from build123d import *

# Parameters (mm, degrees)
F2_DEPTH       = 20
F4_D           = 4
F4_CSINK_D     = 8
F4_CSINK_ANGLE = 90
F6_W           = 8
F6_H           = 2
F7_DEPTH       = 16.001


with BuildPart() as f2:
    # F1 (on Right) → F2 (new body, symmetric)
    with BuildSketch(Plane.YZ):
        Polygon((-16, 0), (0, 0), (0, 16), align=None)
    extrude(amount=F2_DEPTH, both=True)

    # F4 (through all)
    with Locations(Plane(origin=(0, -8, 8), x_dir=(1, 0, 0), z_dir=(0, -0.7071067812, 0.7071067812))):
        with Locations((-12, 0)):
            CounterSinkHole(F4_D / 2, F4_CSINK_D / 2, counter_sink_angle=F4_CSINK_ANGLE)

    # F5: F2 across plane


with BuildPart() as f2_1:
    add(f2.part)
    add(f2.part.mirror(Plane.YZ), mode=Mode.INTERSECT)

    # F6 (on face) → F7 (cut, through all)
    with BuildSketch(Plane(origin=(0, 0, 0), x_dir=(1, 0, 0), z_dir=(0, 0, -1))):
        with Locations((0, 1)):
            Rectangle(F6_W, F6_H)
    extrude(amount=-F7_DEPTH, mode=Mode.SUBTRACT)


solid = f2_1.part
Verification items for the finished model (mm, model axes). A direction names the side the tool comes from. Coordinates: 2 decimals unless noted, no trailing zeros. Order: outer loops, then holes, each group sorted by start corner. A loop starts at its lowest first (then second) coordinate and runs counter-clockwise, first axis right, second up. Notation, with made-up numbers: M 85.25,-25.5 L 128.25,-25.5 A25 cw 128.25,7.5 Z; hole C 42.25,64.25 d9. An arc over 180 degrees is marked long. One line per item, written item: value. Start each with the question number.
Item 1: Sectioned sample at A-A (z = 15). Enter the section's corners in (x, y), then the cut area to 3 significant figures.
Item 2: Access from +Z, -Z, +X, -X, +Y, -Y to the whole of each face (thin tool, end or side, straight path). Record for faces 1 (the flat face through (20, -5, 5)), 2 (the flat face through (4, -1, 8)).
Item 3: Sectioned sample at C-C (x = -12). Enter the section's corners in (y, z).
Item 4: Sectioned sample at B-B (z = 13.25). Enter the section's corners in (x, y).
Item 5: Mould release check, pull along X, two halves, no side actions. Record for faces 3 (the flat face through (12, 0, 8)), 4 (the cylindrical face through (10, -4, 4)), 5 (the flat face through (-20, -5, 5)): released by +X, released by -X, zero draft, split by the parting line, or undercut.
Item 6: Gauge pin test, flat ends, axial feed: pin 1 (8 mm diameter, centred on x = -4.5, z = 13.5, fed in from +Y); pin 2 (2 mm diameter, centred on x = -3.5, z = 5.5, fed in from -Y); pin 3 (2 mm diameter, centred on x = -0.5, y = -5, fed in from +Z); pin 4 (4 mm diameter, centred on x = 0.5, z = 4, fed in from +Y). Record the tip position at first contact, or that the pin passes through.
Item 7: Sectioned sample at D-D (z = 4.5). Count the separate pieces of the cut face and the enclosed holes in it, then the cut area to 3 significant figures.
Item 8: Scan lines: probe 1 along X at (y, z) = (-1.25, 8); probe 2 along X at (y, z) = (-3, 4); probe 3 along Y at (x, z) = (-1, 2). Record each from-to range of solid material in increasing order.
Conclusion:
1. outline: M -20,-1 L -4,-1 L -4,0 L -20,0 Z; M 4,-1 L 20,-1 L 20,0 L 4,0 Z
1. area: 32.0 mm^2
2. face 1: +Z, -Z, +X, +Y, -Y
2. face 2: +Z, -Z, +Y
3. outline: M -16,0 L -2.83,0 L -8,5.17 L -10.83,5.17 Z; M -5.17,8 L 0,2.83 L 0,16 L -5.17,10.83 Z
4. outline: M -20,-2.75 L 20,-2.75 L 20,0 L 4,0 L 4,-2 L -4,-2 L -4,0 L -20,0 Z
5. face 3: zero draft
5. face 4: undercut
5. face 5: released by -X
6. pin 1: stops at y = 0
6. pin 2: stops at y = -11.5
6. pin 3: stops at z = 12
6. pin 4: stops at y = -2
7. separate pieces: 1
7. enclosed holes: 2
7. area: 408 mm^2
8. probe 1: x = -20 to -4, 4 to 20
8. probe 2: x = -20 to -13.87, -10.13 to 10.13, 13.87 to 20
8. probe 3: y = -14 to -2
